from build123d import *

# Parameters (mm, degrees)
SKETCH_1_W                 = 52
SKETCH_1_H                 = 47
EXTRUDE_1_DEPTH            = 9
SKETCH_19_R                = 23.75
SKETCH_19_R_2              = 12
CUT_EXTRUDE_2_DEPTH        = 2
SKETCH_20_R                = 5
EXTRUDE_3_DEPTH            = 4.4
SKETCH_21_R                = 4
EXTRUDE_4_DEPTH            = 6
SKETCH_22_R                = 8
CUT_EXTRUDE_5_DEPTH        = 39
CUT_EXTRUDE_6_DEPTH        = 47
HOLE_WIZARD_M3_1_D         = 2.5
HOLE_WIZARD_M3_1_DEPTH     = 9.5
HOLE_WIZARD_M3_1_TIP       = 0.751075774
HOLE_WIZARD_M4_2_D         = 3.3
HOLE_WIZARD_M4_2_DEPTH     = 10.1
HOLE_WIZARD_M4_2_TIP       = 0.991420021
CHAMFER_3_SIZE             = 0.5
CHAMFER_6_SIZE             = 2
EXTRUDE3_DEPTH             = 2
EXTRUDE4_REACH             = 57.474
SKETCH_35_R                = 3.25
CUT_EXTRUDE_1_DEPTH        = 2
PATTERN_CIRCULAR_1_COUNT   = 3
HOLE_WIZARD_2_AT_2_COUNT   = 2
HOLE_WIZARD_2_AT_2_PITCH   = 19.052558883
HOLE_WIZARD_2_AT_3_COUNT   = 2
HOLE_WIZARD_2_AT_3_PITCH   = 19.052558883
HOLE_WIZARD_M3_2_D         = 2.5
HOLE_WIZARD_M3_2_DEPTH     = 7.5
HOLE_WIZARD_M3_2_TIP       = 0.751075774
CUT_EXTRUDE_START          = 10
CUT_EXTRUDE_3_DEPTH        = 10
SKETCH_42_R                = 2
CUT_EXTRUDE_4_DEPTH        = 2
CHAMFER_7_SIZE             = 0.5
SKETCH_43_R                = 1
CUT_EXTRUDE_5_2_DEPTH      = 5
SKETCH_44_R                = 2.75
CUT_EXTRUDE_7_DEPTH        = 2
HOLE_WIZARD_2_2_AT_2_COUNT = 2
HOLE_WIZARD_2_2_AT_2_PITCH = 35
SKETCH_46_R                = 2.25
CUT_EXTRUDE_8_DEPTH        = 3
SKETCH_48_W                = 2.005209087
SKETCH_48_H                = 2.691311543
SKETCH_48_W_2              = 2.943459277
SKETCH_48_H_2              = 3.25
CUT_EXTRUDE_9_DEPTH        = 2
CUT_EXTRUDE_START_2        = 7
CUT_EXTRUDE_12_DEPTH       = 7
CUT_EXTRUDE_13_OUTLINE_R   = 2.75
CUT_EXTRUDE_13_DEPTH       = 5
CUT_EXTRUDE_START_3        = -0.7
CUT_EXTRUDE_13_2_DEPTH     = 0.7


# Read off the part's stored shape, not the designer's step: 切除-拉伸13
with BuildPart() as part:
    # 草图1 → 拉伸1 (new body)
    with BuildSketch(Plane.XY):
        Rectangle(SKETCH_1_W, SKETCH_1_H)
    extrude(amount=EXTRUDE_1_DEPTH)

    # 草图19 → Cut-Extrude 2 (cut)
    with BuildSketch(Plane.XY.offset(9)):
        with Locations((0, -4)):
            Circle(SKETCH_19_R)
        with Locations((0, -4)):
            Circle(SKETCH_19_R_2, mode=Mode.SUBTRACT)
    extrude(amount=-CUT_EXTRUDE_2_DEPTH, mode=Mode.SUBTRACT)

    # 草图20 → 拉伸3 (add)
    with BuildSketch(Plane.XY.offset(9)):
        with Locations((0, -4)):
            Circle(SKETCH_20_R)
    extrude(amount=EXTRUDE_3_DEPTH)

    # 草图21 → 拉伸4 (add)
    with BuildSketch(Plane.XY.offset(13.4)):
        with Locations((0, -4)):
            Circle(SKETCH_21_R)
    extrude(amount=EXTRUDE_4_DEPTH)

    # 草图22 → Cut-Extrude 5 (cut, symmetric)
    with BuildSketch(Plane.XY.offset(9)):
        with Locations((11, 0.795831523)):
            Circle(SKETCH_22_R)
    extrude(amount=CUT_EXTRUDE_5_DEPTH, both=True, mode=Mode.SUBTRACT)

    # 草图25 → 拉伸6 (cut)
    with BuildSketch(Plane.XZ.offset(23.5)):
        Polygon((-26, 8), (-14.574815946, 0), (-26, 0), align=None)
    extrude(amount=-CUT_EXTRUDE_6_DEPTH, mode=Mode.SUBTRACT)

    # M3 螺纹孔1
    with Locations(Plane(origin=(-11, 23.5, 3.5), x_dir=(0, 0, 1), z_dir=(0, 1, 0))):
        with Locations((0, 0), (0, 30)):
            Hole(HOLE_WIZARD_M3_1_D / 2, depth=HOLE_WIZARD_M3_1_DEPTH)
            with Locations((0, 0, -(HOLE_WIZARD_M3_1_DEPTH + HOLE_WIZARD_M3_1_TIP / 2))):  # 118° drill point
                Cone(0, HOLE_WIZARD_M3_1_D / 2, HOLE_WIZARD_M3_1_TIP, mode=Mode.SUBTRACT)

    # M4 螺纹孔2
    with Locations(Plane(origin=(0, -4, 19.4), x_dir=(1, 0, 0), z_dir=(0, 0, 1))):
        with Locations((0, 0)):
            Hole(HOLE_WIZARD_M4_2_D / 2, depth=HOLE_WIZARD_M4_2_DEPTH)
            with Locations((0, 0, -(HOLE_WIZARD_M4_2_DEPTH + HOLE_WIZARD_M4_2_TIP / 2))):  # 118° drill point
                Cone(0, HOLE_WIZARD_M4_2_D / 2, HOLE_WIZARD_M4_2_TIP, mode=Mode.SUBTRACT)

    # 倒角3
    chamfer_3_edges = [part.edges().sort_by_distance(p)[0] for p in [
        (-4, -4, 19.4),
        (1.65, -4, 19.4),
    ]]
    chamfer(chamfer_3_edges, length=CHAMFER_3_SIZE)

    # 倒角6
    chamfer_6_edges = [part.edges().sort_by_distance(p)[0] for p in [
        (26, 23.5, 4.5),
    ]]
    chamfer(chamfer_6_edges, length=CHAMFER_6_SIZE)

    # Sketch6 → Extrude3 (cut)
    with BuildSketch(Plane.XZ.offset(23.5)):
        Polygon((-26, 9), (-26, 8), (-14.574815946, 0), (26, 0), (26, 9), (13.557746863, 9), (13.557746863, 7), (-13.557746863, 7), (-13.557746863, 9), align=None)
    extrude(amount=-EXTRUDE3_DEPTH, mode=Mode.SUBTRACT)

    # Extrude4: up to this face of the body (flat: up to its plane)
    extrude4_end = Plane(part.part.faces().sort_by_distance((1.330613504, 23.5, 4.737278788))[0])
    # Sketch7 → Extrude4 (cut, up to the picked face)
    with BuildSketch(Plane.XZ.offset(21.5), mode=Mode.PRIVATE) as extrude4_sk1:
        Polygon((-20, 9), (-20, 6), (-11.43111196, 0), (-14.574815946, 0), (-26, 8), (-26, 9), align=None)
    extrude4_tool1 = split(extrude(extrude4_sk1.sketch, amount=-EXTRUDE4_REACH, mode=Mode.PRIVATE), bisect_by=extrude4_end, keep=Keep.BOTH, mode=Mode.PRIVATE)
    add(extrude4_tool1.solids().sort_by(Axis((-19.659359, -21.5, 5.073959), (0, 1, 0)))[0], mode=Mode.SUBTRACT)

    # 草图35 → 切除-拉伸1 (cut)
    with BuildSketch(Plane.XY.offset(9)):
        with Locations((1.473720558, 6.295831523)):
            Circle(SKETCH_35_R)
    cut_extrude_1 = extrude(amount=-CUT_EXTRUDE_1_DEPTH, mode=Mode.SUBTRACT)

    # 阵列(圆周)1: 切除-拉伸1 ×3 about axis
    pattern_circular_1_axis = Axis((11, 0.795831523, 0), (0, 0, 1))
    for i in range(1, PATTERN_CIRCULAR_1_COUNT):
        add(cut_extrude_1.rotate(pattern_circular_1_axis, i * 360 / PATTERN_CIRCULAR_1_COUNT), mode=Mode.SUBTRACT)

    # 草图36 → Hole Wizard 2 (revolve, cut)
    with BuildSketch(Plane(origin=(1.473720558, 6.295831523, 7), x_dir=(0, -1, 0), z_dir=(1, 0, 0))):
        Polygon((0, 0), (0, 7), (1.5, 7), (1.5, 3.7), (3.5, 3.7), (3.5, 0), align=None)
    hole_wizard_2 = revolve(axis=Axis((1.473720558, 6.295831523, 13.35), (0, 0, -1)), mode=Mode.SUBTRACT)

    # Hole Wizard 2 at 2: Hole Wizard 2 ×2
    with Locations(*[(i * HOLE_WIZARD_2_AT_2_PITCH, 0, 0) for i in range(1, HOLE_WIZARD_2_AT_2_COUNT)]):
        add(hole_wizard_2, mode=Mode.SUBTRACT)

    # Hole Wizard 2 at 3: Hole Wizard 2 ×2
    with Locations(*[Vector(0.49999999999999806, -0.8660254037844398, 0) * (i * HOLE_WIZARD_2_AT_3_PITCH) for i in range(1, HOLE_WIZARD_2_AT_3_COUNT)]):
        add(hole_wizard_2, mode=Mode.SUBTRACT)

    # M3 螺纹孔2
    with Locations(Plane(origin=(-11, -21.5, 3.5), x_dir=(0, 0, -1), z_dir=(0, -1, 0))):
        with Locations((0, 0), (0, 35)):
            Hole(HOLE_WIZARD_M3_2_D / 2, depth=HOLE_WIZARD_M3_2_DEPTH)
            with Locations((0, 0, -(HOLE_WIZARD_M3_2_DEPTH + HOLE_WIZARD_M3_2_TIP / 2))):  # 118° drill point
                Cone(0, HOLE_WIZARD_M3_2_D / 2, HOLE_WIZARD_M3_2_TIP, mode=Mode.SUBTRACT)

    # 草图41 → 切除-拉伸3 (cut)
    with BuildSketch(Plane.XY.offset(7).offset(CUT_EXTRUDE_START)):
        with BuildLine():
            Line((1.473720558, 9.795831523), (7.585559388, 9.795831523))
            ThreePointArc((7.585559388, 9.795831523), (11.085559388, 6.295831523), (7.585559388, 2.795831523))
            Line((7.585559388, 2.795831523), (1.473720558, 2.795831523))
            ThreePointArc((1.473720558, 2.795831523), (-2.026279442, 6.295831523), (1.473720558, 9.795831523))
        make_face()
    extrude(amount=-CUT_EXTRUDE_3_DEPTH, mode=Mode.SUBTRACT)

    # 草图42 → 切除-拉伸4 (cut)
    with BuildSketch(Plane(origin=(0, 0, 0), x_dir=(-1, 0, 0), z_dir=(0, 0, -1))):
        with Locations((6, 18.295831523)):
            Circle(SKETCH_42_R)
        with Locations((6, -16.704168477)):
            Circle(SKETCH_42_R)
    extrude(amount=-CUT_EXTRUDE_4_DEPTH, mode=Mode.SUBTRACT)

    # 倒角7
    chamfer_7_edges = [part.edges().sort_by_distance(p)[0] for p in [
        (-4, 18.295831523, 0),
        (-4, -16.704168477, 0),
    ]]
    chamfer(chamfer_7_edges, length=CHAMFER_7_SIZE)

    # 草图43 → Cut-Extrude 5 2 (cut)
    with BuildSketch(Plane(origin=(0, 0, 2), x_dir=(-1, 0, 0), z_dir=(0, 0, -1))):
        with Locations((6, 18.295831523)):
            Circle(SKETCH_43_R)
        with Locations((6, -16.704168477)):
            Circle(SKETCH_43_R)
    extrude(amount=-CUT_EXTRUDE_5_2_DEPTH, mode=Mode.SUBTRACT)

    # 草图44 → 切除-拉伸7 (cut)
    with BuildSketch(Plane.XY.offset(9)):
        with Locations((-6, 18.295831523)):
            Circle(SKETCH_44_R)
    extrude(amount=-CUT_EXTRUDE_7_DEPTH, mode=Mode.SUBTRACT)

    # 草图45 → Hole Wizard 2 2 (revolve, cut)
    with BuildSketch(Plane(origin=(-6, 18.295831523, 7), x_dir=(0, -1, 0), z_dir=(1, 0, 0))):
        Polygon((0, 0), (0, 7), (1, 7), (1, 3), (2.5, 3), (2.5, 0), align=None)
    hole_wizard_2_2 = revolve(axis=Axis((-6, 18.295831523, 13.35), (0, 0, -1)), mode=Mode.SUBTRACT)

    # Hole Wizard 2 2 at 2: Hole Wizard 2 2 ×2
    with Locations(*[(0, -i * HOLE_WIZARD_2_2_AT_2_PITCH, 0) for i in range(1, HOLE_WIZARD_2_2_AT_2_COUNT)]):
        add(hole_wizard_2_2, mode=Mode.SUBTRACT)

    # 草图46 → 切除-拉伸8 (cut)
    with BuildSketch(Plane.XY.offset(7)):
        with Locations((-6, -16.704168477)):
            Circle(SKETCH_46_R)
    extrude(amount=CUT_EXTRUDE_8_DEPTH, mode=Mode.SUBTRACT)

    # 草图48 → 切除-拉伸9 (cut)
    with BuildSketch(Plane.XY.offset(9)):
        Polygon((-20, -21.5), (-16.056540723, -21.5), (-20, -16.808688457), align=None)
        with Locations((-18.997395457, 10.154344229)):
            Rectangle(SKETCH_48_W, SKETCH_48_H)
        with Locations((17.528270361, -19.875)):
            Rectangle(SKETCH_48_W_2, SKETCH_48_H_2)
    extrude(amount=-CUT_EXTRUDE_9_DEPTH, mode=Mode.SUBTRACT)

    # 草图52 → 切除-拉伸12 (cut)
    with BuildSketch(Plane.XY.offset(3.3).offset(CUT_EXTRUDE_START_2)):
        with BuildLine():
            Line((7.5, -10.204168477), (7.5, 0.795831523))
            ThreePointArc((7.5, 0.795831523), (11, 4.295831523), (14.5, 0.795831523))
            Line((14.5, 0.795831523), (14.5, -10.204168477))
            ThreePointArc((14.5, -10.204168477), (11, -13.704168477), (7.5, -10.204168477))
        make_face()
    extrude(amount=-CUT_EXTRUDE_12_DEPTH, mode=Mode.SUBTRACT)

    # 切除-拉伸13 outline → 切除-拉伸13 (cut)
    with BuildSketch(Plane.XY.offset(4)):
        with BuildLine():
            Line((18.979967897, 1.361616253), (22.276279442, 3.26474261))
            ThreePointArc((22.276279442, 3.26474261), (23.557368355, 8.045831523), (18.776279442, 9.326920437))
            Line((18.776279442, 9.326920437), (15.479967897, 7.423794079))
            ThreePointArc((15.479967897, 7.423794079), (17.92820323, 4.795831523), (18.979967897, 1.361616253))
        make_face()
        with BuildLine():
            ThreePointArc((4.964881512, 6.047245127), (5.697596566, 6.786200278), (6.520032103, 7.423794079))
            Line((6.520032103, 7.423794079), (3.223720558, 9.326920437))
            ThreePointArc((3.223720558, 9.326920437), (4.56508103, 7.937017202), (4.964881512, 6.047245127))
        make_face()
        with BuildLine():
            Line((-0.276279442, 3.26474261), (3.020032103, 1.361616253))
            ThreePointArc((3.020032103, 1.361616253), (3.160986763, 2.392663221), (3.43458317, 3.396690647))
            ThreePointArc((3.43458317, 3.396690647), (1.598092305, 2.798041983), (-0.276279442, 3.26474261))
        make_face()
        with Locations((-6, -16.704168477)):
            Circle(CUT_EXTRUDE_13_OUTLINE_R)
    extrude(amount=CUT_EXTRUDE_13_DEPTH, mode=Mode.SUBTRACT)

    # Cut-Extrude 13 2 outline → Cut-Extrude 13 2 (cut)
    with BuildSketch(Plane.XY.offset(4).offset(CUT_EXTRUDE_START_3)):
        with BuildLine():
            Line((18.979967897, 1.361616253), (22.276279442, 3.26474261))
            ThreePointArc((22.276279442, 3.26474261), (20.401907695, 2.798041983), (18.56541683, 3.396690647))
            ThreePointArc((18.56541683, 3.396690647), (18.839013237, 2.392663221), (18.979967897, 1.361616253))
        make_face()
        with BuildLine():
            ThreePointArc((17.035118488, 6.047245127), (17.43491897, 7.937017202), (18.776279442, 9.326920437))
            Line((18.776279442, 9.326920437), (15.479967897, 7.423794079))
            ThreePointArc((15.479967897, 7.423794079), (16.302403434, 6.786200278), (17.035118488, 6.047245127))
        make_face()
        with BuildLine():
            ThreePointArc((4.964881512, 6.047245127), (5.697596566, 6.786200278), (6.520032103, 7.423794079))
            Line((6.520032103, 7.423794079), (3.223720558, 9.326920437))
            ThreePointArc((3.223720558, 9.326920437), (4.56508103, 7.937017202), (4.964881512, 6.047245127))
        make_face()
        with BuildLine():
            Line((-0.276279442, 3.26474261), (3.020032103, 1.361616253))
            ThreePointArc((3.020032103, 1.361616253), (3.160986763, 2.392663221), (3.43458317, 3.396690647))
            ThreePointArc((3.43458317, 3.396690647), (1.598092305, 2.798041983), (-0.276279442, 3.26474261))
        make_face()
    extrude(amount=CUT_EXTRUDE_13_2_DEPTH, mode=Mode.SUBTRACT)


solid = part.part
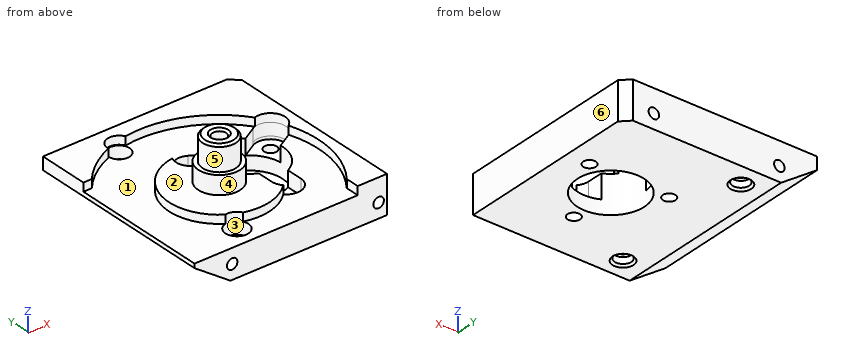
Design review of the part built by this model. Coordinates are the model's own, in mm. Face numbers are marked on the shaded views. A direction names the side the tool comes from. Coordinates: 2 decimals unless noted, no trailing zeros. Order: outer loops, then holes, each group sorted by start corner. A loop starts at its lowest first (then second) coordinate and runs counter-clockwise, first axis right, second up. Notation, with made-up numbers: (-40, 64) -> (-24, 64) arc R29 cw to (-24, 90) -> close; hole circle Ø6 at (79, 51). An arc over 180 degrees is marked (long way). Use one line per item in the form item = value. Start each with the question number.
(1) Add section C-C on z = 17.5. State the section outline as (x, y) points, plus the area to 3 significant figures.
(2) For the marked faces 5 and 6, list the 3-axis set-ups (+Z, -Z, +X, -X, +Y, -Y) from which the entire face can be reached by the end or side of a thin tool; tool diameter is ignored.
(3) The part is to be moulded in two halves that separate along X. For the marked faces 1, 2, 3 and 4, say which applies: +X half, -X half, draft (parallel to the pull), parting line (faces both ways), or undercut.
(4) Add section B-B on y = 10.5. State the section outline as (x, z) points, plus the area to 3 significant figures.
(5) For probe 1 along Y at (x, z) = (11, 1.8); probe 2 along Y at (x, z) = (-6, 1.4); probe 3 along Z at (x, y) = (19, 20.75), list the stretches that pass through material, from the lowest coordinate up.
(6) Insertion check: pin 1 (1 mm diameter, centred on y = 4.5, z = 11, fed in from -X); pin 2 (4 mm diameter, centred on x = -7, y = 18.5, fed in from +Z); pin 3 (0.6 mm diameter, centred on y = -19.5, z = 8, fed in from -X); pin 4 (5.5 mm diameter, centred on x = 12, y = -9.5, fed in from +Z). Each pin has a flat end and moves straight along its axis. Give the tip position at first contact, or say it passes through.
(7) Add section A-A on x = -17. State the section outline as (y, z) points (3 decimals), plus the area to 3 significant figures.
Answer block:
q1.outline = circle Ø8 at (0, -4); hole circle Ø3.3 at (0, -4)
q1.area = 41.7 mm²
q2.face_5 = +Z
q2.face_6 = +Z, -Z, +X, +Y, -Y
q3.face_1 = undercut
q3.face_2 = draft
q3.face_3 = undercut
q3.face_4 = parting line
q4.outline = (-20, 6) -> (-11.43, 0) -> (26, 0) -> (26, 9) -> (18.81, 9) -> (18.81, 7) -> (-20, 7) -> close
q4.area = 311 mm²
q5.probe_1 = -21.5 to -11.7, -8.7 to -7.2, 8.8 to 23.5
q5.probe_2 = -21.5 to -18.7, -14.7 to 16.3, 20.3 to 23.5
q5.probe_3 = 0 to 2.25, 4.75 to 9
q6.pin_1 = through
q6.pin_2 = 9
q6.pin_3 = 19
q6.pin_4 = 7
q7.outline = (-21.5, 3.899) -> (23.5, 3.899) -> (23.5, 9) -> (12.585, 9) -> (12.585, 7) -> (-21.5, 7) -> close
q7.area = 161 mm²
